Read the model definition and answer for the solid it produces. Units are mm, in the model's axes. A direction names the side the tool comes from. Round coordinates to 2 decimals unless told otherwise and drop trailing zeros. Order: outer loops, then holes, each group sorted by start corner. A loop starts at its lowest first (then second) coordinate and runs counter-clockwise, first axis right, second up. Notation, with made-up numbers: (37.25, 83) - (51.25, 83) arc R33 cw to (51.25, 112) - close; hole circle Ø7 at (55.5, 43). An arc over 180 degrees is marked (long way). Answer as a JSON object with one key per item and string values. Group by question number.
Q1. A cutting plane is placed at D-D on y = 37.5. Determine the outline of the cut face in (x, z).
Q2. Given pin 1 Ø6 at (x, z) = (39, -2) entering from -Y; pin 2 Ø6 at (x, y) = (115, 7) entering from -Z; pin 3 Ø6 at (x, y) = (116.5, -5) entering from +Z, each flat-ended and moving along its own axis, determine where each tip first touches the part or whether it passes through.
Q3. Consider line 1 (Y direction, x = 110, z = 1); line 2 (X direction, y = 0, z = -2); line 3 (X direction, y = 30, z = -57.5). Determine where each line is inside the solid, lowest interval first.
Q4. A cutting plane is placed at C-C on x = 88. Determine the outline of the cut face in (y, z).
Q5. A cutting plane is placed at A-A on x = 110. Determine the outline of the cut face in (y, z), and give its area (3 significant figures).
Q6. A cutting plane is placed at B-B on z = 0. Determine the outline of the cut face in (x, y).
Q7. The mould has two halves that part along X. Classify faces 4 (the cylindrical face through (103.759, -0.26, 11.064)), 5 (the cylindrical face through (106.116, 0.957, -0.131)), 6 (the cylindrical face through (5.07, -9.764, -74.362)): pulls with the +X half, pulls with the -X half, needs draft (parallel to the pull), parting line crosses it, or undercut.
Q8. A tool of negligible diameter and unlimited length cuts with its end or side. For faces 1 (the cylindrical face through (59.589, 19.076, -6.007)), 2 (the flat face through (116, 0, 7.5)), 3 (the flat face through (116, 0, -7.5)), from which of +Z, -Z, +X, -X, +Y, -Y can it reach the whole face along a straight path? Write none if from no direction.
```python
from build123d import *

# Parameters (mm, degrees)
CUT_EXTRUDE1_DEPTH      = 20
FILLET1_R               = 12.5
CUT_EXTRUDE2_DEPTH      = 164.802472582
CUT_EXTRUDE2_DEPTH_BACK = 164.802472582
SKETCH3_R               = 4


with BuildPart() as part:
    # Sketch1 → Revolve1 (revolve)
    with BuildSketch(Plane.XY):
        with BuildLine():
            Line((0, 0), (0, 75))
            Line((0, 75), (10, 75))
            Line((10, 75), (10, 34))
            ThreePointArc((10, 34), (10.585786438, 32.585786438), (12, 32))
            Line((12, 32), (18, 32))
            ThreePointArc((18, 32), (19.414213562, 31.414213562), (20, 30))
            Line((20, 30), (20, 20))
            Line((20, 20), (120, 20))
            Line((120, 20), (120, 0))
            Line((120, 0), (10, 0))
            Line((10, 0), (0, 0))
        make_face()
    revolve(axis=Axis((120, 0, 0), (-1, 0, 0)))

    # Sketch2 → Cut-Extrude1 (cut)
    with BuildSketch(Plane(origin=(120, 0, 0), x_dir=(0, 0, -1), z_dir=(1, 0, 0))):
        with BuildLine():
            Line((-7.5, 18.540496218), (-7.5, -18.540496218))
            ThreePointArc((-7.5, -18.540496218), (-20, 0), (-7.5, 18.540496218))
        make_face()
        with BuildLine():
            Line((7.5, 18.540496218), (7.5, -18.540496218))
            ThreePointArc((7.5, -18.540496218), (20, 0), (7.5, 18.540496218))
        make_face()
    extrude(amount=-CUT_EXTRUDE1_DEPTH, mode=Mode.SUBTRACT)

    # Fillet1
    fillet1_edges = [part.edges().sort_by_distance(p)[0] for p in [
        (100, 0, -7.5),
        (100, 0, 7.5),
    ]]
    fillet(fillet1_edges, radius=FILLET1_R - 0.0001)  # a hair under: the kernel refuses the full size

    # Sketch3 → Cut-Extrude2 (cut, two sides: drawn at the far end of the back side and taken through both)
    with BuildSketch(Plane.XY.offset(7.5).offset(-CUT_EXTRUDE2_DEPTH_BACK)):
        with Locations(Location((110, 0, 0), (0, 0, 308.682187453))):
            Circle(SKETCH3_R)
    extrude(amount=CUT_EXTRUDE2_DEPTH + CUT_EXTRUDE2_DEPTH_BACK, mode=Mode.SUBTRACT)


solid = part.part
```
Result set:
{
 "1": {"outline": "(0, -64.95) - (10, -64.95) - (10, 64.95) - (0, 64.95) - close"},
 "2": {"pin 1": "stops at y = -20", "pin 2": "stops at z = -7.51", "pin 3": "stops at z = 7.5"},
 "3": {"line 1": "y = -19.97 to -4, 4 to 19.97", "line 2": "x = 0 to 106, 114 to 120", "line 3": "x = 0 to 10"},
 "4": {"outline": "circle Ø40 at (0, 0)"},
 "5": {"outline": "(-18.44, -7.75) - (-4, -7.75) - (-4, 7.75) - (-18.44, 7.75) arc R20 ccw to start; (4, -7.75) - (18.44, -7.75) arc R20 ccw to (18.44, 7.75) - (4, 7.75) - close", "area": "480 mm²"},
 "6": {"outline": "(0, -75) - (10, -75) - (10, -34) arc R2 cw to (12, -32) - (18, -32) arc R2 ccw to (20, -30) - (20, -20) - (120, -20) - (120, 20) - (20, 20) - (20, 30) arc R2 ccw to (18, 32) - (12, 32) arc R2 cw to (10, 34) - (10, 75) - (0, 75) - close; hole circle Ø8 at (110, 0)"},
 "7": {"face 4": "pulls with the +X half", "face 5": "undercut", "face 6": "needs draft"},
 "8": {"face 1": "+X", "face 2": "+Z, +X, +Y, -Y", "face 3": "-Z, +X, +Y, -Y"}
}
